Design review of the part shown in the three views and the two pictorial views. Dimensions are in mm from the part's minimum x, y and z. Round coordinates to 2 decimals unless told otherwise and drop trailing zeros. Order: outer loops, then holes, each group sorted by start corner. A loop starts at its lowest first (then second) coordinate and runs counter-clockwise, first axis right, second up. Notation, with made-up numbers: M 24,79.5 L 70,79.5 A7 ccw 70,90.5 Z; hole C 21.5,45 d11. An arc over 180 degrees is marked long. Use a Markdown table: item, result. Add a question column.
(1) Take a section at B-B (z = 20). Write out the cut boundary in (x, y).
(2) For pin 1 (3 mm diameter, centred on x = 40.5, y = 9.5, fed in from -Z); pin 2 (1 mm diameter, centred on y = 4.5, z = 17, fed in from -X); pin 3 (7.5 mm diameter, centred on y = 5.5, z = 16, fed in from +X), all flat-tipped, find the tip position at first contact; note any pin that passes through.
(3) To check wall thickness, follow probe 1 along Y at (x, z) = (185, 24); probe 2 along X at (y, z) = (8.25, 31.5); probe 3 along X at (y, z) = (9.25, 23). State the ranges of each line that lie inside material, in increasing order. Write a range as from..to.
(4) Take a section at A-A (y = 8). Write out the cut boundary in (x, z), then the cut area to 3 significant figures.
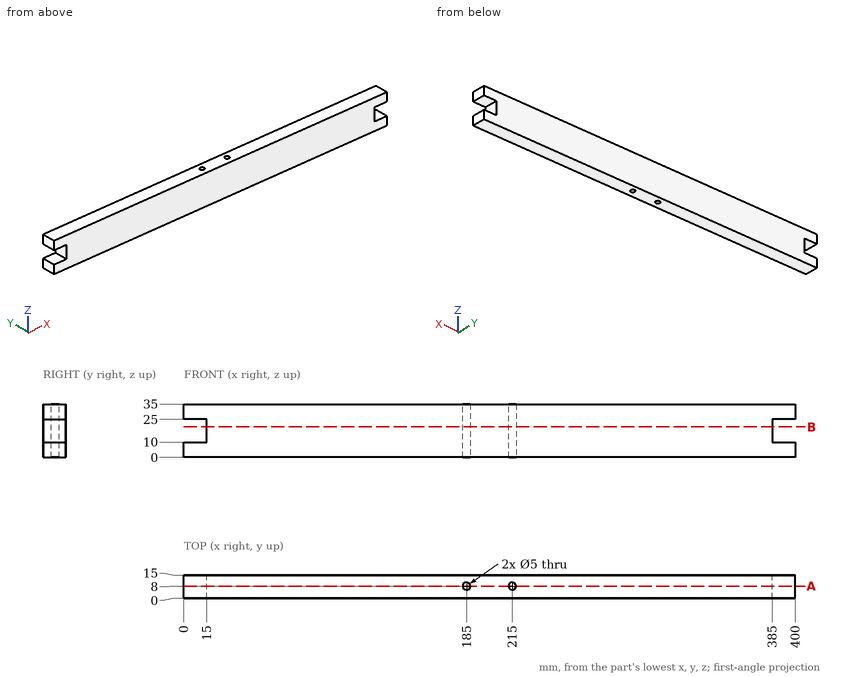
Verdict:
| question | item | result |
|---|---|---|
| 1 | outline | M 15,0 L 385,0 L 385,15 L 15,15 Z; hole C 185,8 d5; hole C 215,8 d5 |
| 2 | pin 1 | stops at z = 0 |
| 2 | pin 2 | stops at x = 15 |
| 2 | pin 3 | stops at x = 385 |
| 3 | probe 1 | y = 0..5.5, 10.5..15 |
| 3 | probe 2 | x = 0..182.51, 187.49..212.51, 217.49..400 |
| 3 | probe 3 | x = 15..182.83, 187.17..212.83, 217.17..385 |
| 4 | outline | M 0,0 L 182.5,0 L 182.5,35 L 0,35 L 0,25 L 15,25 L 15,10 L 0,10 Z; M 187.5,0 L 212.5,0 L 212.5,35 L 187.5,35 Z; M 217.5,0 L 400,0 L 400,10 L 385,10 L 385,25 L 400,25 L 400,35 L 217.5,35 Z |
| 4 | area | 13,200 mm^2 |
